Autodesk Inventor part; units mm, degrees
ref_plane "YZ Plane" through (0, 0, 0) normal (1, 0, 0) x (0, 1, 0)
ref_plane "XZ Plane" through (0, 0, 0) normal (0, 1, 0) x (-1, 0, 0)
ref_plane "XY Plane" through (0, 0, 0) normal (0, 0, 1) x (1, 0, 0)
sketch "スケッチ1" plane through (0, 0, 0) normal (1, 0, 0) x (0, 1, 0)
  line L0 (125.6523, 179.1954) -> (-474.3477, 179.1954)
  line L1 (-474.3477, 179.1954) -> (-474.3477, -102.8046)
  line L2 (-474.3477, -102.8046) -> (125.6523, -102.8046)
  line L3 (125.6523, -102.8046) -> (125.6523, 179.1954)
  dimension "d0" = 600
  dimension "d1" = 282
extrude "押し出し1" add sketch "スケッチ1" along normal blind 2.6
sketch "スケッチ4" plane through (2.6, 0, 0) normal (1, 0, 0) x (0, 0, -1)
  line L0 (102.8046, 125.6523) -> (-179.1954, 125.6523)
  line L1 (-179.1954, 125.6523) -> (-179.1954, -474.3477)
  point P0 (0, 0)
  point P1 (-139.1954, -225.3477)
  point P2 (-139.1954, -123.3477)
  dimension "d19" = 102
  dimension "d20" = 249
  dimension "d21" = 40
  dimension "d22" = 40
hole "穴2" at (2.6, -225.3477, 139.1954) at (2.6, -123.3477, 139.1954) direction (-1, 0, 0) diameter 6.6 end through all
sketch "スケッチ5" plane through (2.6, 0, 0) normal (1, 0, 0) x (0, 0, -1)
  line L0 (-179.1954, 125.6523) -> (-179.1954, -474.3477)
  line L1 (102.8046, 125.6523) -> (-179.1954, 125.6523)
  point P0 (-152.1954, -84.3477)
  dimension "d30" = 27
  dimension "d31" = 210
hole "穴3" at (2.6, -84.3477, 152.1954) direction (-1, 0, 0) diameter 18 end through all
sketch "スケッチ6" plane through (2.6, 0, 0) normal (1, 0, 0) x (0, 0, -1)
  line L0 (-179.1954, 125.6523) -> (-179.1954, -474.3477)
  circle A0 centre (-152.1954, -84.3477) radius 9
  point P0 (0, 0)
  point P1 (-166.6954, -53.9477)
  point P2 (-151.6954, -53.9477)
  dimension "d39" = 12.5
  dimension "d40" = 27.5
  dimension "d41" = 30.4
  dimension "d42" = 30.4
hole "穴4" at (2.6, -53.9477, 166.6954) at (2.6, -53.9477, 151.6954) direction (-1, 0, 0) diameter 4.5 end through all
sketch "スケッチ7" plane through (2.6, 0, 0) normal (1, 0, 0) x (0, 0, -1)
  line L0 (102.8046, 125.6523) -> (-179.1954, 125.6523)
  line L1 (102.8046, -474.3477) -> (102.8046, 125.6523)
  line L2 (-179.1954, -474.3477) -> (102.8046, -474.3477)
  point P0 (0, 0)
  point P1 (84.0046, -56.9477)
  point P2 (84.0046, -291.9477)
  dimension "d50" = 182.6
  dimension "d51" = 18.8
  dimension "d52" = 18.8
  dimension "d53" = 182.4
hole "穴5" at (2.6, -56.9477, -84.0046) at (2.6, -291.9477, -84.0046) direction (-1, 0, 0) diameter 6.7 end through all
sketch "スケッチ8" plane through (2.6, 0, 0) normal (1, 0, 0) x (0, 0, -1)
  line L0 (102.8046, -474.3477) -> (102.8046, 125.6523)
  line L1 (102.8046, 125.6523) -> (107.8046, 125.6523)
  line L2 (117.7603, -23.9477) -> (102.8046, -23.9477)
  line L3 (102.8046, -89.9477) -> (117.7603, -89.9477)
  line L4 (107.8046, 125.6523) -> (107.8046, -474.3477)
  line L5 (107.8046, -474.3477) -> (102.8046, -474.3477)
  line L6 (102.8046, -258.9477) -> (107.8046, -258.9477)
  line L7 (102.8046, -324.9477) -> (107.8046, -324.9477)
  circle A0 centre (84.0046, -56.9477) radius 3.35
  circle A1 centre (84.0046, -291.9477) radius 3.35
  point P0 (0, 0)
  point P1 (107.8046, -23.9477)
  point P2 (107.8046, -89.9477)
  dimension "d61" = 5
  dimension "d62" = 33
  dimension "d63" = 33
  dimension "d64" = 33
  dimension "d65" = 33
extrude "押し出し3" add sketch "スケッチ8" against normal blind 2.6 contours L0 L7 L4 L5 | L0 L3 L4 L6 | L0 L1 L4 L2
sketch "スケッチ9" plane through (2.6, 0, 0) normal (1, 0, 0) x (0, 0, -1)
  ellipse E0 centre (-2.4593, 110.6523) end of major axis (-2.4593, 125.1521) minor radius 14.4996 (5.606, 98.6026) -> (5.606, 122.702) ccw
  line L0 (4.4935, 123.5363) -> (-99.9579, 123.5363)
  line L1 (-99.9579, 97.7683) -> (4.4935, 97.7683)
  ellipse E1 centre (-67.383, 110.6523) end of major axis (-67.383, 123.067) minor radius 12.4145 (-70.683, 122.6204) -> (-70.683, 98.6842) ccw
  line L2 (-70.683, 122.6204) -> (-70.683, 125.6523)
  line L3 (102.8046, 125.6523) -> (-179.1954, 125.6523)
  line L4 (5.7266, 122.6204) -> (5.7266, 125.6523)
  line L5 (5.7266, 125.6523) -> (-70.683, 125.6523)
  line L6 (6.1243, 98.9661) -> (4.4935, 97.7683)
  line L7 (-70.683, 98.6842) -> (-66.6998, 97.7683)
  point P0 (0, 0)
extrude "押し出し4" cut sketch "スケッチ9" against normal blind 3
properties part number "lc_box_side" material "ポリカーボネート、クリア"
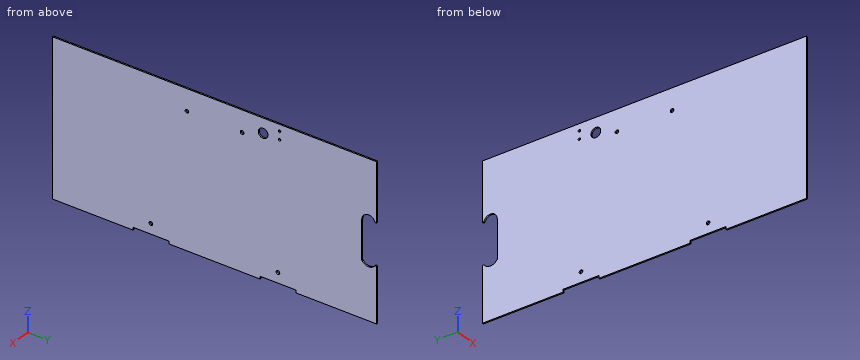
Model file for the job. Use its own axes, mm. Give positions to 0.01 mm unless a question says otherwise; leave off trailing zeros. Order: outer loops, then holes, each group sorted by start corner. A loop starts at its lowest first (then second) coordinate and runs counter-clockwise, first axis right, second up. Notation, with made-up numbers: (-20, -6.75) - (29, -6.75) arc R31 cw to (29, 26.25) - close; hole circle Ø6 at (-26, 72.25). An arc over 180 degrees is marked (long way). One line per item, written item: value.
Item 1: Wall check: line 1 (Y direction, x = 2.35, z = 152); line 2 (Y direction, x = 1.25, z = -10); line 3 (Y direction, x = 1.8, z = 54). Give the ranges that are in metal, low to high.
Response values:
line 1: -474.35 to -93.35, -75.35 to -56.18, -51.72 to 125.65
line 2: -474.35 to 103.24, 118.07 to 125.65
line 3: -474.35 to 97.77
Item 2: Slice it at C-C (x = 0.65). Give the number of separate pieces and of enclosed holes in the cut face, then the cut area to 3 significant figures.
Response values:
separate pieces: 1
enclosed holes: 7
area: 169,000 mm2
Item 3: Pin check, flat tip, straight feed: pin 1 Ø6 at (y, z) = (-56.95, -84) entering from -X. Stop position of the tip, or through.
Response values:
pin 1: through
Item 4: Slice it at A-A (y = -268). List the corners of the cut face in (x, z), then the cut area to 3 significant figures.
Response values:
outline: (0, -102.8) - (2.6, -102.8) - (2.6, 179.2) - (0, 179.2) - close
area: 733 mm2
Item 5: Slice it at B-B (z = 19). List the corners of the cut face in (x, y), then the cut area to 3 significant figures.
Response values:
outline: (0, -474.35) - (2.6, -474.35) - (2.6, 97.77) - (0, 97.77) - close
area: 1,490 mm2
